Study the drawing (mm; zero at the part's minimum x, y, z) and answer. A direction names the side the tool comes from. Give positions to 0.01 mm unless a question says otherwise; leave off trailing zeros. Write each loop counter-clockwise with the first axis right and the second up, starting at its lowest first coordinate (ties: lowest second). Pieces come first, ordered by that corner, then holes. Notation, with made-up numbers: M 22.25,-14 L 60.25,-14 A17 cw 60.25,-8 Z; hole C 80,52 d11. An arc over 180 degrees is marked long. Use a Markdown table: item, result. Add a question column.
Item 1: For the marked faces 5 and 6, determine the directions among +Z, -Z, +X, -X, +Y, -Y from which every point of the face is accessible in a straight line to the end or side of a thin tool.
Item 2: A cutting plane is placed at C-C on z = 84. Determine the outline of the cut face in (x, y).
Item 3: The mould has two halves that part along X. Classify the marked faces 1, 2, 3 and 4: pulls with the +X half, pulls with the -X half, needs draft (parallel to the pull), parting line crosses it, or undercut.
Item 4: A cutting plane is placed at A-A on y = 36. Determine the outline of the cut face in (x, z).
Item 5: Given P1, Ø10, axis at x = 14.5, z = 40.5, coming from the +Y side; P2, Ø12, axis at x = 55.5, z = 89, coming from the +Y side, each flat-ended and moving along its own axis, determine where each tip first touches the part or whether it passes through.
Item 6: Consider probe 1 along Z at (x, y) = (51, 28); probe 2 along X at (y, z) = (37, 92); probe 3 along Y at (x, z) = (23, 70). Determine where each line is inside the solid, lowest interval first. Write a range as [from, to].
Item 7: A cutting plane is placed at B-B on x = 14. Determine the outline of the cut face in (y, z).
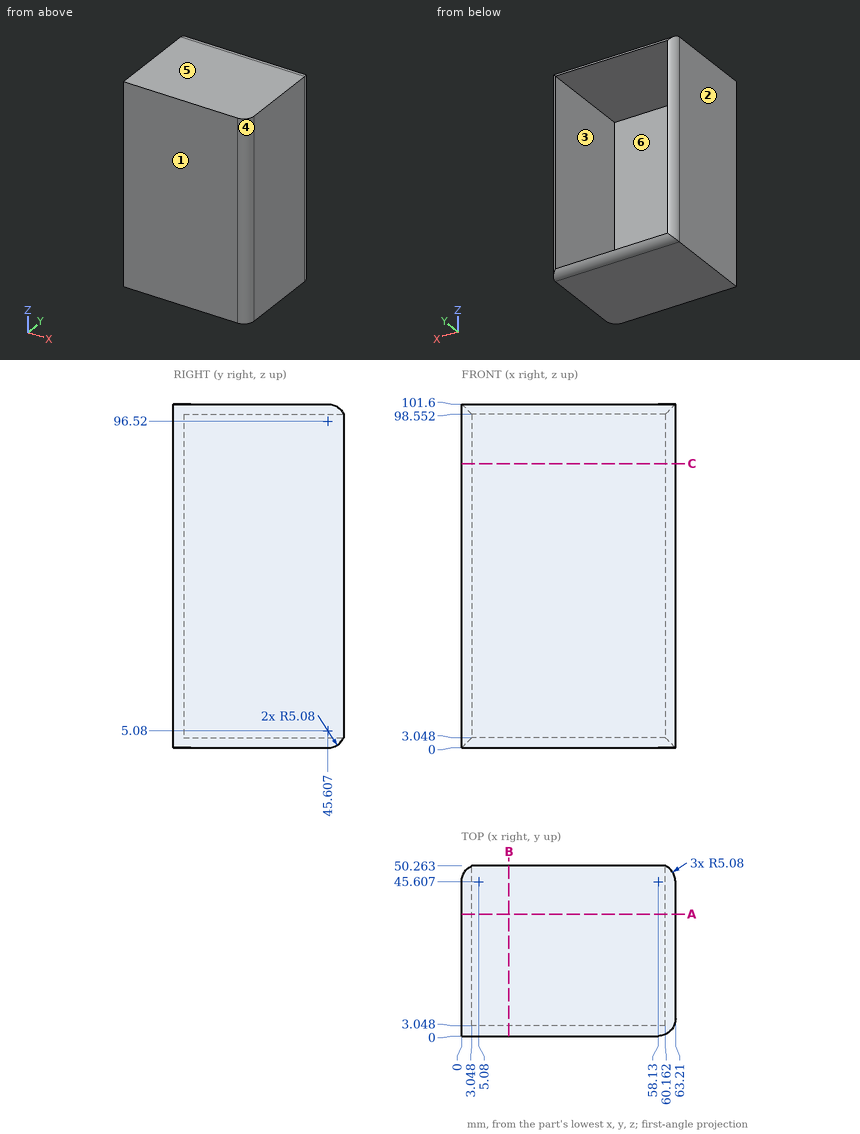
Filled in:
| question | item | result |
|---|---|---|
| 1 | face 5 | +Z, +X, -X, +Y, -Y |
| 1 | face 6 | +Y |
| 2 | outline | M 0,0 L 58.13,0 A5.08 ccw 63.21,5.08 L 63.21,45.61 A5.08 ccw 60.16,50.26 L 60.16,3.05 L 3.05,3.05 L 3.05,50.26 A5.08 ccw 0,45.61 Z |
| 3 | face 1 | needs draft |
| 3 | face 2 | pulls with the -X half |
| 3 | face 3 | undercut |
| 3 | face 4 | pulls with the +X half |
| 4 | outline | M 0,0 L 63.21,0 L 63.21,101.6 L 0,101.6 Z; hole M 3.05,3.05 L 60.16,3.05 L 60.16,98.55 L 3.05,98.55 Z |
| 5 | P1 | y = 3.05 |
| 5 | P2 | y = 50.26 |
| 6 | probe 1 | [0, 3.05], [98.55, 101.6] |
| 6 | probe 2 | [0, 3.05], [60.16, 63.21] |
| 6 | probe 3 | [0, 3.05] |
| 7 | outline | M 0,0 L 45.61,0 A5.08 ccw 50.26,3.05 L 3.05,3.05 L 3.05,98.55 L 50.26,98.55 A5.08 ccw 45.61,101.6 L 0,101.6 Z |
